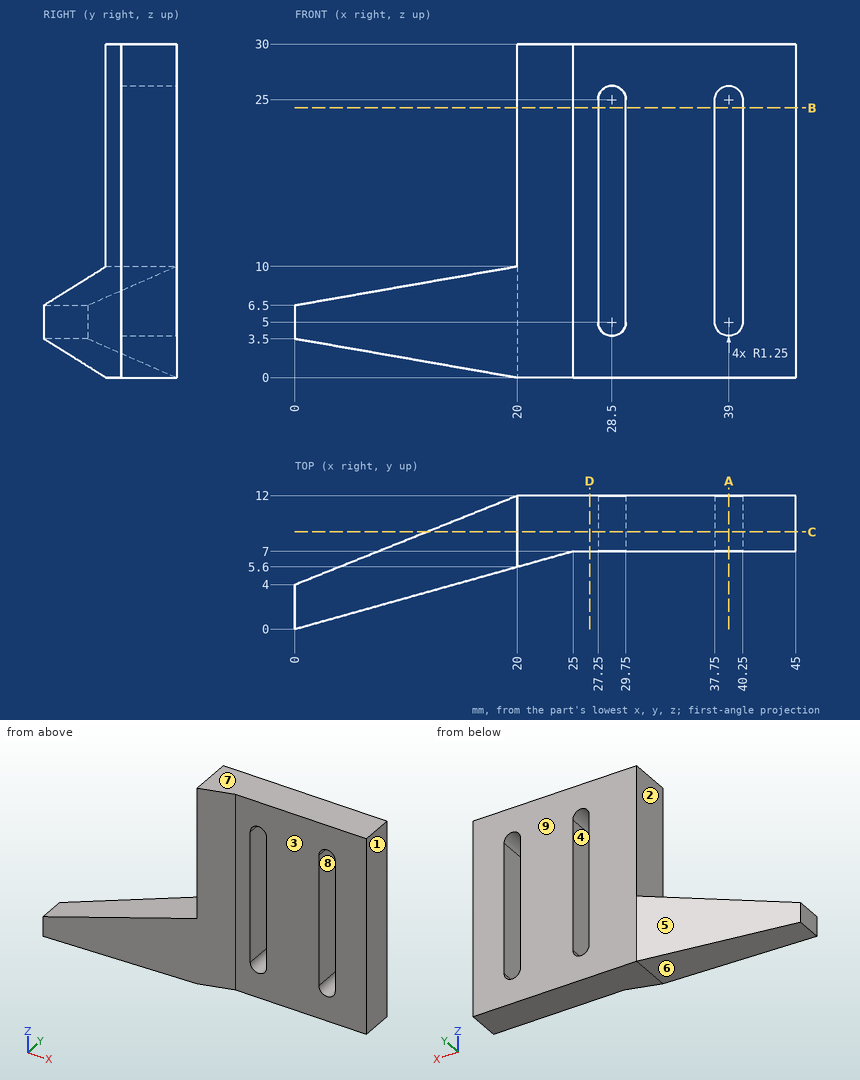
Part print with two shaded views. Sizes in mm from the minimum x, y, z corner. A direction names the side the tool comes from. Round coordinates to 2 decimals unless told otherwise and drop trailing zeros. Loops run counter-clockwise (first coordinate to the right, second up) from the corner with the lowest first, then second, coordinate; pieces in that order, holes last. Notation, with made-up numbers: M 76.5,-5.5 L 92.5,-5.5 A13 ccw 92.5,17.5 Z; hole C 63.5,-2 d4. An arc over 180 degrees is marked long. Return JSON: item names as keys, results as strings. Group by question number.
(1) Drop flat-ended pins along their axis: P1, Ø2.5, axis at y = 8.5, z = 19.5, coming from the -X side; P2, Ø1.5, axis at x = 32.5, z = 22.5, coming from the -Y side; P3, Ø6, axis at y = 4.5, z = 6.5, coming from the +X side. Give the stop position or say it passes through.
(2) Tool access for the marked faces 1, 2, 3, 4 and 5: list every direction of +Z, -Z, +X, -X, +Y, -Y with a clear straight run to the whole face (end or side of a thin tool).
(3) Saw through at D-D, the plane x = 26.5. List the corners of the cut face in (y, z), and give its area (3 significant figures).
(4) Mould opens along Z. For the marked faces 6, 7, 8 and 9 say: +Z half, -Z half, draft (parallel to the pull), parting line (faces both ways), or undercut.
(5) Saw through at A-A, the plane x = 39. List the corners of the cut face in (y, z).
(6) Saw through at B-B, the plane z = 24.25. List the corners of the cut face in (x, y), and give its area (4 significant figures).
(7) Saw through at C-C, the plane y = 8.75. List the corners of the cut face in (x, z) (3 decimals), and give its area (3 significant figures).
(8) Wall check: probe 1 along X at (y, z) = (8.5, 22.5); probe 2 along X at (y, z) = (11.5, 5.5); probe 3 along Y at (x, z) = (38, 27.25). Give the ranges that are in metal, low to high. Write a range as [from, to].
Answer list:
{
 "1": {"P1": "x = 20", "P2": "y = 7", "P3": "x = 45"},
 "2": {"face 1": "+Z, -Z, +X, +Y, -Y", "face 2": "+Z, -X, +Y, -Y", "face 3": "+Z, -Z, +X, -Y", "face 4": "+Y, -Y", "face 5": "+Z, -Z, -X, +Y"},
 "3": {"outline": "M 7,0 L 12,0 L 12,30 L 7,30 Z", "area": "150 mm2"},
 "4": {"face 6": "-Z half", "face 7": "+Z half", "face 8": "undercut", "face 9": "draft"},
 "5": {"outline": "M 7,0 L 12,0 L 12,3.75 L 7,3.75 Z; M 7,26.25 L 12,26.25 L 12,30 L 7,30 Z"},
 "6": {"outline": "M 20,5.6 L 25,7 L 27.25,7 L 27.25,12 L 20,12 Z; M 29.75,7 L 37.75,7 L 37.75,12 L 29.75,12 Z; M 40.25,7 L 45,7 L 45,12 L 40.25,12 Z", "area": "103.5 mm2"},
 "7": {"outline": "M 11.875,1.422 L 20,0 L 45,0 L 45,30 L 20,30 L 20,10 L 11.875,8.578 Z; hole M 27.25,5 A1.25 ccw 29.75,5 L 29.75,25 A1.25 ccw 27.25,25 Z; hole M 37.75,5 A1.25 ccw 40.25,5 L 40.25,25 A1.25 ccw 37.75,25 Z", "area": "710 mm2"},
 "8": {"probe 1": "[20, 27.25], [29.75, 37.75], [40.25, 45]", "probe 2": "[18.75, 27.25], [29.75, 37.75], [40.25, 45]", "probe 3": "[7, 12]"}
}
